```python
from build123d import *

# Parameters (mm, degrees)
F1_DEPTH  = 35
F3_DEPTH  = 33
F5_R      = 4
F6_DEPTH  = 16.2
F4_R      = 2.25
F7_DEPTH  = 25
F8_R      = 3.55
F9_DEPTH  = 3
F10_R     = 4.65
F11_DEPTH = 5
F12_R     = 5


with BuildPart() as f1:
    # F0 (on Top) → F1 (new body)
    with BuildSketch(Plane.XY):
        with BuildLine():
            Line((39, 33.6), (-39, 33.6))
            ThreePointArc((-39, 33.6), (-42.5355339059, 32.1355339059), (-44, 28.6))
            Line((-44, 28.6), (-44, -28.6))
            ThreePointArc((-44, -28.6), (-42.5355339059, -32.1355339059), (-39, -33.6))
            Line((-39, -33.6), (39, -33.6))
            ThreePointArc((39, -33.6), (42.5355339059, -32.1355339059), (44, -28.6))
            Line((44, -28.6), (44, 28.6))
            ThreePointArc((44, 28.6), (42.5355339059, 32.1355339059), (39, 33.6))
        make_face()
        with BuildLine():
            ThreePointArc((-41.65, 26.15), (-40.1855339059, 29.6855339059), (-36.65, 31.15))
            Line((-36.65, 31.15), (36.65, 31.15))
            ThreePointArc((36.65, 31.15), (40.1855339059, 29.6855339059), (41.65, 26.15))
            Line((41.65, 26.15), (41.65, -26.15))
            ThreePointArc((41.65, -26.15), (40.1855339059, -29.6855339059), (36.65, -31.15))
            Line((36.65, -31.15), (-36.65, -31.15))
            ThreePointArc((-36.65, -31.15), (-40.1855339059, -29.6855339059), (-41.65, -26.15))
            Line((-41.65, -26.15), (-41.65, 26.15))
        make_face(mode=Mode.SUBTRACT)
        with BuildLine():
            Line((36.65, 31.15), (-36.65, 31.15))
            ThreePointArc((-36.65, 31.15), (-40.1855339059, 29.6855339059), (-41.65, 26.15))
            Line((-41.65, 26.15), (-41.65, -26.15))
            ThreePointArc((-41.65, -26.15), (-40.1855339059, -29.6855339059), (-36.65, -31.15))
            Line((-36.65, -31.15), (36.65, -31.15))
            ThreePointArc((36.65, -31.15), (40.1855339059, -29.6855339059), (41.65, -26.15))
            Line((41.65, -26.15), (41.65, 26.15))
            ThreePointArc((41.65, 26.15), (40.1855339059, 29.6855339059), (36.65, 31.15))
        make_face()
    extrude(amount=F1_DEPTH)

    # F2 (on Top) → F3 (cut)
    with BuildSketch(Plane.XY):
        with BuildLine():
            ThreePointArc((41.65, 26.15), (40.1855339059, 29.6855339059), (36.65, 31.15))
            Line((36.65, 31.15), (-36.65, 31.15))
            ThreePointArc((-36.65, 31.15), (-40.1855339059, 29.6855339059), (-41.65, 26.15))
            Line((-41.65, 26.15), (-41.65, -26.15))
            ThreePointArc((-41.65, -26.15), (-40.1855339059, -29.6855339059), (-36.65, -31.15))
            Line((-36.65, -31.15), (36.65, -31.15))
            ThreePointArc((36.65, -31.15), (40.1855339059, -29.6855339059), (41.65, -26.15))
            Line((41.65, -26.15), (41.65, 26.15))
        make_face()
    extrude(amount=F3_DEPTH, mode=Mode.SUBTRACT)

    # F5 (on face) → F6 (join)
    with BuildSketch(Plane.XY.offset(35)):
        with Locations((-32, 24.6)):
            Circle(F5_R)
        with Locations((12, 24.6)):
            Circle(F5_R)
        with Locations((-32, -24.6)):
            Circle(F5_R)
        with Locations((12, -24.6)):
            Circle(F5_R)
    extrude(amount=-F6_DEPTH)

    # F4 (on face) → F7 (cut)
    with BuildSketch(Plane.XY.offset(35)):
        with Locations((-32, 24.6)):
            Circle(F4_R)
        with Locations((-32, -24.6)):
            Circle(F4_R)
        with Locations((12, 24.6)):
            Circle(F4_R)
        with Locations((12, -24.6)):
            Circle(F4_R)
    extrude(amount=-F7_DEPTH, mode=Mode.SUBTRACT)

    # F8 (on face) → F9 (cut)
    with BuildSketch(Plane.XY.offset(35)):
        with Locations((-32, 24.6)):
            Circle(F8_R)
        with Locations((12, 24.6)):
            Circle(F8_R)
        with Locations((12, -24.6)):
            Circle(F8_R)
        with Locations((-32, -24.6)):
            Circle(F8_R)
    extrude(amount=-F9_DEPTH, mode=Mode.SUBTRACT)

    # F10 (on face) → F11 (cut)
    with BuildSketch(Plane(origin=(-44, 0, 0), x_dir=(0, -1, 0), z_dir=(-1, 0, 0))):
        with Locations((0, 25)):
            Circle(F10_R)
    extrude(amount=-F11_DEPTH, mode=Mode.SUBTRACT)

    # F12
    f12_edges = [f1.edges().sort_by_distance(p)[0] for p in [
        (0, 33.6, 35),
    ]]
    fillet(f12_edges, radius=F12_R)


solid = f1.part
```
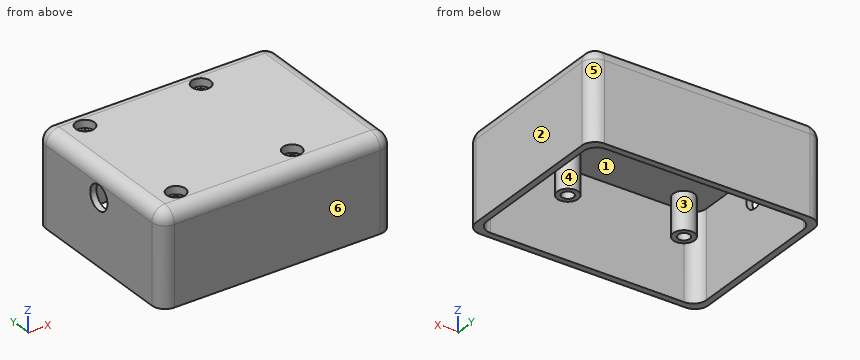
Model file for the job. Use its own axes, mm. Face numbers are marked on the shaded views. A direction names the side the tool comes from. Coordinates: 2 decimals unless noted, no trailing zeros. Order: outer loops, then holes, each group sorted by start corner. A loop starts at its lowest first (then second) coordinate and runs counter-clockwise, first axis right, second up. Notation, with made-up numbers: (-40, 75) -> (-12, 75) arc R13 ccw to (-12, 84) -> close; hole circle Ø11 at (84.25, -28). An arc over 180 degrees is marked (long way). Answer as a JSON object with one key per item and string values. Group by question number.
1) Cut at D-D, the plane y = 0. Write the cut outline in (x, z), then the cut area to 3 significant figures.
2) Drill centre lines: L1, parallel to Y at x = 12, z = 23; L2, parallel to X at y = -8, z = 11; L3, parallel to Y at x = 10, z = 23.5. Where is each one in solid material? Low to high.
3) Flat gauge pins, fed straight in: pin 1 (4 mm diameter, centred on x = -1, y = -21, fed in from -Z); pin 2 (5 mm diameter, centred on x = -32, y = 24.6, fed in from -Z); pin 3 (7 mm diameter, centred on x = 12, y = -24.6, fed in from +Z); pin 4 (4 mm diameter, centred on x = 12, y = 24.6, fed in from -Z). Where does each tip first touch, or does it go through?
4) Cut at A-A, the plane z = 25. Count the separate pieces of the cut face and the enclosed holes in it, then the cut area to 3 significant figures.
5) Which spindle directions (+Z, -Z, +X, -X, +Y, -Y) get a long thin tool onto all of the face, cutting with end or side? Do the marked faces 1 and 2. Say none if no direction does.
6) Pull direction X, two halves, no side cores. Call the marked faces 3, 4, 5 and 6: +X half, -X half, draft (parallel to the pull), parting line (faces both ways), or undercut.
Check values:
{
 "1": {"outline": "(-44, 0) -> (-41.65, 0) -> (-41.65, 20.35) -> (-44, 20.35) -> close; (-44, 29.65) -> (-41.65, 29.65) -> (-41.65, 33) -> (41.65, 33) -> (41.65, 0) -> (44, 0) -> (44, 30) arc R5 ccw to (39, 35) -> (-39, 35) arc R5 ccw to (-44, 30) -> close", "area": "299 mm²"},
 "2": {"L1": "y = -33.6 to -31.15, -28.6 to -26.85, -22.35 to -20.6, 20.6 to 22.35, 26.85 to 28.6, 31.15 to 33.6", "L2": "x = -44 to -41.65, 41.65 to 44", "L3": "y = -33.6 to -31.15, -28.06 to -25.63, -23.57 to -21.14, 21.14 to 23.57, 25.63 to 28.06, 31.15 to 33.6"},
 "3": {"pin 1": "stops at z = 33", "pin 2": "stops at z = 18.8", "pin 3": "stops at z = 32", "pin 4": "passes through"},
 "4": {"separate pieces": "5", "enclosed holes": "4", "area": "840 mm²"},
 "5": {"face 1": "-Z", "face 2": "+Z, -Z, +X, +Y, -Y"},
 "6": {"face 3": "undercut", "face 4": "undercut", "face 5": "+X half", "face 6": "draft"}
}
